Input: part model. Units: mm. Frame: model coordinates. Give positions to 0.01 mm unless a question says otherwise; leave off trailing zeros. Loops run counter-clockwise (first coordinate to the right, second up) from the corner with the lowest first, then second, coordinate; pieces in that order, holes last. Notation, with made-up numbers: M -30,67 L 13,67 A21 ccw 13,89 Z; hole C 77,25 d9. An arc over 180 degrees is marked long. Answer as a JSON object with one key per item and string values. Group by question number.
1) First-contact query: P1, Ø5, axis at x = 25, z = 1.5, coming from the +Y side; P2, Ø5, axis at x = -101.5, z = 4.5, coming from the -Y side; P3, Ø5, axis at y = 16.5, z = 6.5, coming from the -X side; P4, Ø1, axis at x = 104.5, z = 3.5, coming from the +Y side. Flat tips, straight axial feed; report the tip coordinate or a pass-through.
2) Ray query, L1, parallel to Y at x = -125, z = 8; L2, parallel to Y at x = -57.5, z = 1.75; L3, parallel to X at y = 40, z = 4.25. Return the intervals inside material, ascending.
3) Section query A-A on x = -66. Return loops of the section in (y, z).
4) Draft query along X for faces 1 (the flat face through (-180, 5, 6)), 2 (the flat face through (174, 10, 6)), 3 (the flat face through (-161.2, 298, 6)). Return one class per face: +X half, -X half, draft (parallel to the pull), parting line (faces both ways), or undercut.
5) Section query C-C on y = 71. Return loops of the section in (x, z).
6) Section query B-B on z = 10.5. Count the separate pieces of the cut face and the enclosed holes in it, plus the area to 3 significant figures.
from build123d import *

# Parameters (mm, degrees)
SKETCH1_R           = 5
SKETCH1_R_2         = 11
SKETCH1_R_3         = 3
SKETCH1_R_4         = 4
SKETCH1_R_5         = 0.8
SKETCH1_W           = 12.4
SKETCH1_H           = 10
SKETCH1_W_2         = 50
SKETCH1_H_2         = 12.4
SKETCH1_H_3         = 30
SKETCH1_W_3         = 20
BOSS_EXTRUDE1_DEPTH = 12.4


with BuildPart() as part:
    # Sketch1 → Boss-Extrude1 (new body)
    with BuildSketch(Plane.XY):
        with BuildLine():
            Line((-180, 0), (180, 0))
            Line((180, 0), (180, 10))
            Line((180, 10), (167.6, 10))
            Line((167.6, 10), (167.6, 20))
            Line((167.6, 20), (180, 20))
            Line((180, 20), (180, 30))
            ThreePointArc((180, 30), (24.399116368, 178.368906186), (-35.000570148, 385.000570148))
            Line((-35.000570148, 385.000570148), (-40, 390))
            Line((-40, 390), (-140, 390))
            Line((-140, 390), (-150, 390))
            Line((-150, 390), (-180, 360))
            Line((-180, 360), (-180, 30))
            Line((-180, 30), (-180, 20))
            Line((-180, 20), (-167.6, 20))
            Line((-167.6, 20), (-167.6, 10))
            Line((-167.6, 10), (-180, 10))
            Line((-180, 10), (-180, 0))
        make_face()
        with Locations(Location((-151.2, 319.2, 0), (0, 0, 180))):
            Circle(SKETCH1_R, mode=Mode.SUBTRACT)
        with Locations(Location((-90, 298, 0), (0, 0, 180))):
            Circle(SKETCH1_R_2, mode=Mode.SUBTRACT)
        with Locations(Location((-90, 323, 0), (0, 0, 180))):
            Circle(SKETCH1_R_3, mode=Mode.SUBTRACT)
        with Locations(Location((-90, 368, 0), (0, 0, 180))):
            Circle(SKETCH1_R_4, mode=Mode.SUBTRACT)
        with Locations(Location((-90, 375, 0), (0, 0, 180))):
            Circle(SKETCH1_R_5, mode=Mode.SUBTRACT)
        with Locations(Location((-90, 361, 0), (0, 0, 180))):
            Circle(SKETCH1_R_5, mode=Mode.SUBTRACT)
        with Locations(Location((-90, 221, 0), (0, 0, 180))):
            Circle(SKETCH1_R_5, mode=Mode.SUBTRACT)
        with Locations(Location((-90, 228, 0), (0, 0, 180))):
            Circle(SKETCH1_R_4, mode=Mode.SUBTRACT)
        with Locations(Location((-90, 235, 0), (0, 0, 180))):
            Circle(SKETCH1_R_5, mode=Mode.SUBTRACT)
        with Locations(Location((-90, 273, 0), (0, 0, 180))):
            Circle(SKETCH1_R_3, mode=Mode.SUBTRACT)
        with Locations(Location((-48.8, 15, 0), (0, 0, 180))):
            Circle(SKETCH1_R, mode=Mode.SUBTRACT)
        with Locations((65, 15)):
            Rectangle(SKETCH1_W, SKETCH1_H, mode=Mode.SUBTRACT)
        with Locations((0, 15)):
            Rectangle(SKETCH1_W, SKETCH1_H, mode=Mode.SUBTRACT)
        with Locations((-65, 15)):
            Rectangle(SKETCH1_W, SKETCH1_H, mode=Mode.SUBTRACT)
        with Locations((102.5, 36.2)):
            Rectangle(SKETCH1_W_2, SKETCH1_H_2, mode=Mode.SUBTRACT)
        with Locations((0, 36.2)):
            Rectangle(SKETCH1_W_2, SKETCH1_H_2, mode=Mode.SUBTRACT)
        with Locations((-102.5, 36.2)):
            Rectangle(SKETCH1_W_2, SKETCH1_H_2, mode=Mode.SUBTRACT)
        with Locations((-120, 298)):
            Rectangle(SKETCH1_W, SKETCH1_H_3, mode=Mode.SUBTRACT)
        with Locations((-120, 343)):
            Rectangle(SKETCH1_W, SKETCH1_H_3, mode=Mode.SUBTRACT)
        with Locations((-120, 253)):
            Rectangle(SKETCH1_W, SKETCH1_H_3, mode=Mode.SUBTRACT)
        with Locations((-151.2, 340.4)):
            Rectangle(SKETCH1_W_3, SKETCH1_H_2, mode=Mode.SUBTRACT)
        with Locations((-151.2, 298)):
            Rectangle(SKETCH1_W_3, SKETCH1_H_2, mode=Mode.SUBTRACT)
        with Locations((-151.2, 255.6)):
            Rectangle(SKETCH1_W_3, SKETCH1_H_2, mode=Mode.SUBTRACT)
        with Locations((-53.4, 358)):
            Rectangle(SKETCH1_W, SKETCH1_H_3, mode=Mode.SUBTRACT)
        with Locations((-53.4, 298)):
            Rectangle(SKETCH1_W, SKETCH1_H_3, mode=Mode.SUBTRACT)
        with Locations((-53.4, 238)):
            Rectangle(SKETCH1_W, SKETCH1_H_3, mode=Mode.SUBTRACT)
        with Locations((-53.4, 178)):
            Rectangle(SKETCH1_W, SKETCH1_H_3, mode=Mode.SUBTRACT)
    extrude(amount=BOSS_EXTRUDE1_DEPTH)


solid = part.part
Output:
{
 "1": {"P1": "stops at y = 181.54", "P2": "stops at y = 0", "P3": "stops at x = -167.6", "P4": "stops at y = 83.12"},
 "2": {"L1": "y = 0 to 30, 42.4 to 238, 268 to 283, 313 to 328, 358 to 390", "L2": "y = 0 to 163, 193 to 223, 253 to 283, 313 to 343, 373 to 390", "L3": "x = -180 to -127.5, -77.5 to -25, 25 to 77.5, 127.5 to 162.59"},
 "3": {"outline": "M 0,0 L 10,0 L 10,12.4 L 0,12.4 Z; M 20,0 L 390,0 L 390,12.4 L 20,12.4 Z"},
 "4": {"face 1": "-X half", "face 2": "draft", "face 3": "undercut"},
 "5": {"outline": "M -180,0 L 118.38,0 L 118.38,12.4 L -180,12.4 Z"},
 "6": {"separate pieces": "1", "enclosed holes": "27", "area": "78,400 mm^2"}
}
